Work out the finished part from the listing and answer in its coordinate system (mm). Face numbers are marked on the shaded views. A direction names the side the tool comes from. Give positions to 0.01 mm unless a question says otherwise; leave off trailing zeros. Write each loop counter-clockwise with the first axis right and the second up, starting at its lowest first coordinate (ties: lowest second). Pieces come first, ordered by that corner, then holes.
1) Find section A-A (x = 22). Determine the outline of the cut face in (y, z).
2) Find section C-C (y = -33). Determine the outline of the cut face in (x, z).
3) Given pin 1 Ø7 at (x, z) = (-43, 36) entering from +Y; pin 2 Ø8 at (x, y) = (-34, 7) entering from +Z; pin 3 Ø2 at (x, y) = (-1, 41) entering from +Z, each flat-ended and moving along its own axis, determine where each tip first touches the part or whether it passes through.
4) Find section D-D (x = -41.5). Determine the outline of the cut face in (y, z), plus the area to 3 significant figures.
5) Find section B-B (z = 19.5). Determine the outline of the cut face in (x, y).
6) A tool of negligible diameter and unlimited length cuts with its end or side. For the marked faces 5 and 6, from which of +Z, -Z, +X, -X, +Y, -Y can it reach the whole face along a straight path? Write none if from no direction.
7) Determine the mould class of the marked faces 1, 2, 3 and 4 for opening direction X: pulls with the +X half, pulls with the -X half, needs draft (parallel to the pull), parting line crosses it, or undercut.
8) Straight lines are drawn through the part: probe 1 along X at (y, z) = (43.3, 36); probe 2 along Y at (x, z) = (-7, 6); probe 3 along X at (y, z) = (-34, 41). For each, find the intervals that lie inside material, in ascending order.
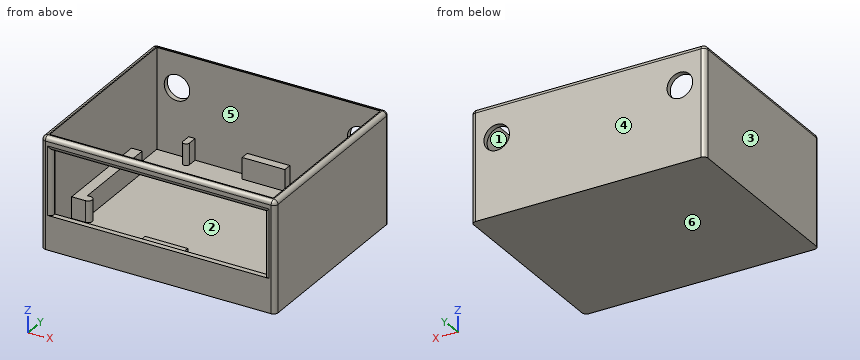
```python
from build123d import *

# Parameters (mm, degrees)
SKETCH_1_W           = 110
SKETCH_1_H           = 90
EXTRUDE_1_DEPTH      = 60
SKETCH_2_W           = 105
SKETCH_2_H           = 85
CUT_EXTRUDE_1_DEPTH  = 55
SKETCH_3_W           = 100
SKETCH_3_H           = 30
CUT_EXTRUDE_2_DEPTH  = 12
SKETCH_4_R           = 6
CUT_EXTRUDE_3_DEPTH  = 12
EXTRUDE_2_DEPTH      = 5
EXTRUDE_2_DEPTH_BACK = 10
SKETCH_6_W           = 20
SKETCH_6_H           = 4
SKETCH_6_W_2         = 5
SKETCH_6_H_2         = 45
EXTRUDE_3_DEPTH      = 5
EXTRUDE_3_DEPTH_BACK = 10
SKETCH_10_W          = 110
SKETCH_10_H          = 8
CUT_EXTRUDE_4_DEPTH  = 122.346610995
FILLET_1_R           = 2


with BuildPart() as part:
    # 스케치1 → 보스-돌출1 (new body)
    with BuildSketch(Plane.XY):
        Rectangle(SKETCH_1_W, SKETCH_1_H)
    extrude(amount=EXTRUDE_1_DEPTH)

    # 스케치2 → 컷-돌출1 (cut)
    with BuildSketch(Plane.XY.offset(60)):
        Rectangle(SKETCH_2_W, SKETCH_2_H)
    extrude(amount=-CUT_EXTRUDE_1_DEPTH, mode=Mode.SUBTRACT)

    # 스케치3 → 컷-돌출2 (cut)
    with BuildSketch(Plane.XZ.offset(45)):
        with Locations((0, 31)):
            Rectangle(SKETCH_3_W, SKETCH_3_H)
    extrude(amount=-CUT_EXTRUDE_2_DEPTH, mode=Mode.SUBTRACT)

    # 스케치4 → 컷-돌출3 (cut)
    with BuildSketch(Plane(origin=(0, 45, 0), x_dir=(1, 0, 0), z_dir=(0, 1, 0))):
        with Locations(Location((-43, -36, 0), (0, 0, 270))):
            Circle(SKETCH_4_R)
        with Locations(Location((43, -36, 0), (0, 0, 270))):
            Circle(SKETCH_4_R)
    extrude(amount=-CUT_EXTRUDE_3_DEPTH, mode=Mode.SUBTRACT)

    # 스케치6 → 보스-돌출2 (add, two sides: drawn at the far end of the back side and taken through both)
    with BuildSketch(Plane.XY.offset(10).offset(-EXTRUDE_2_DEPTH_BACK)):
        with Locations((0, 40.5)):
            Rectangle(SKETCH_6_W, SKETCH_6_H)
        with Locations((50, 0)):
            Rectangle(SKETCH_6_W_2, SKETCH_6_H_2)
        with Locations((0, -40.5)):
            Rectangle(SKETCH_6_W, SKETCH_6_H)
        with Locations((-50, 0)):
            Rectangle(SKETCH_6_W_2, SKETCH_6_H_2)
    extrude(amount=EXTRUDE_2_DEPTH + EXTRUDE_2_DEPTH_BACK)

    # 스케치7 → 보스-돌출3 (add, two sides: drawn at the far end of the back side and taken through both)
    with BuildSketch(Plane.XY.offset(10).offset(-EXTRUDE_3_DEPTH_BACK)):
        with BuildLine():
            Line((-46, -21), (-50, -21))
            Line((-50, -21), (-47.5, -22.5))
            Line((-47.5, -22.5), (-52.5, -22.5))
            Line((-52.5, -22.5), (-52.5, -25))
            Line((-52.5, -25), (-46, -25))
            ThreePointArc((-46, -25), (-44, -23), (-46, -21))
        make_face()
        with BuildLine():
            Line((-34.5, 38), (-34.5, 42.5))
            Line((-34.5, 42.5), (-37.5, 42.5))
            Line((-37.5, 42.5), (-37.5, 38))
            ThreePointArc((-37.5, 38), (-36, 36.5), (-34.5, 38))
        make_face()
        with BuildLine():
            Line((42, -24), (50, -24))
            Line((50, -24), (47.5, -22.5))
            Line((47.5, -22.5), (52.5, -22.5))
            Line((52.5, -22.5), (52.5, -28))
            Line((52.5, -28), (42, -28))
            ThreePointArc((42, -28), (40, -26), (42, -24))
        make_face()
        with BuildLine():
            Line((44.5, 36), (44.5, 42.5))
            Line((44.5, 42.5), (52.5, 42.5))
            Line((52.5, 42.5), (52.5, 28))
            Line((52.5, 28), (44.5, 28))
            ThreePointArc((44.5, 28), (40.5, 32), (44.5, 36))
        make_face()
    extrude(amount=EXTRUDE_3_DEPTH + EXTRUDE_3_DEPTH_BACK)

    # 스케치10 → 컷-돌출4 (cut, through all)
    with BuildSketch(Plane.XZ.offset(45)):
        with Locations((0, 56)):
            Rectangle(SKETCH_10_W, SKETCH_10_H)
    extrude(amount=-CUT_EXTRUDE_4_DEPTH, mode=Mode.SUBTRACT)

    # 필렛1
    fillet_1_edges = [part.edges().sort_by_distance(p)[0] for p in [
        (55, -45, 26),
        (-55, -45, 26),
        (-55, 45, 26),
        (55, 45, 26),
        (0, 45, 52),
        (55, 0, 52),
        (-55, 0, 52),
        (0, -45, 52),
        (50, -45, 31),
        (0, -45, 46),
        (-50, -45, 31),
    ]]
    fillet(fillet_1_edges, radius=FILLET_1_R)


solid = part.part
```
Results:
1. outline: (-45, 0) - (45, 0) - (45, 50) arc R2 ccw to (43, 52) - (42.5, 52) - (42.5, 5) - (-42.5, 5) - (-42.5, 16) - (-45, 16) - close; (-45, 48) arc R2 ccw to (-43, 46) - (-42.5, 46) - (-42.5, 52) - (-43, 52) arc R2 ccw to (-45, 50) - close
2. outline: (-55, 0) - (55, 0) - (55, 50) arc R2 ccw to (53, 52) - (52.5, 52) - (52.5, 5) - (-52.5, 5) - (-52.5, 52) - (-53, 52) arc R2 ccw to (-55, 50) - close
3. pin 1: passes through
3. pin 2: stops at z = 5
3. pin 3: stops at z = 15
4. outline: (-45, 0) - (45, 0) - (45, 30.19) - (42.5, 30.19) - (42.5, 5) - (-42.5, 5) - (-42.5, 16) - (-45, 16) - close; (-45, 48) arc R2 ccw to (-43, 46) - (-42.5, 46) - (-42.5, 52) - (-43, 52) arc R2 ccw to (-45, 50) - close; (42.5, 41.81) - (45, 41.81) - (45, 50) arc R2 ccw to (43, 52) - (42.5, 52) - close
4. area: 578 mm2
5. outline: (-55, -43) arc R2 ccw to (-53, -45) - (-52, -45) arc R2 ccw to (-50, -43) - (-50, -42.5) - (-52.5, -42.5) - (-52.5, 42.5) - (52.5, 42.5) - (52.5, -42.5) - (50, -42.5) - (50, -43) arc R2 ccw to (52, -45) - (53, -45) arc R2 ccw to (55, -43) - (55, 43) arc R2 ccw to (53, 45) - (-53, 45) arc R2 ccw to (-55, 43) - close
6. face 5: +Z
6. face 6: -Z, +X, -X, +Y, -Y
7. face 1: undercut
7. face 2: undercut
7. face 3: pulls with the -X half
7. face 4: needs draft
8. probe 1: x = -54.98 to -49, -37 to 37, 49 to 54.98
8. probe 2: y = -45 to -38.5, 38.5 to 45
8. probe 3: x = -55 to -52.5, 52.5 to 55
